```python
from build123d import *

# Parameters (mm, degrees)
CUT_EXTRUDE1_START = -3.5
CUT_EXTRUDE1_DEPTH = 3.5
SKETCH4_R          = 3.723909236
CUT_EXTRUDE2_DEPTH = 3.5
CUT_EXTRUDE2_DRAFT = -45


with BuildPart() as part:
    # Sketch2 → Revolve1 (revolve)
    with BuildSketch(Plane(origin=(0, 0, 0), x_dir=(0, 0, -1), z_dir=(1, 0, 0))):
        with BuildLine():
            Line((-11.5, 0), (-11.5, 5.604695392))
            ThreePointArc((-11.5, 5.604695392), (-11.491674324, 5.646551392), (-11.467964804, 5.682035196))
            Line((-11.467964804, 5.682035196), (-11.182035196, 5.967964804))
            ThreePointArc((-11.182035196, 5.967964804), (-11.146551392, 5.991674324), (-11.104695392, 6))
            Line((-11.104695392, 6), (-6.032804608, 6))
            ThreePointArc((-6.032804608, 6), (-5.990948608, 5.991674324), (-5.955464804, 5.967964804))
            Line((-5.955464804, 5.967964804), (-5.844535196, 5.857035196))
            ThreePointArc((-5.844535196, 5.857035196), (-5.809051392, 5.833325676), (-5.767195392, 5.825))
            Line((-5.767195392, 5.825), (-4.65, 5.825))
            ThreePointArc((-4.65, 5.825), (-4.543933983, 5.781066017), (-4.5, 5.675))
            Line((-4.5, 5.675), (-4.5, 3.85))
            ThreePointArc((-4.5, 3.85), (-4.397487373, 3.602512627), (-4.15, 3.5))
            Line((-4.15, 3.5), (10.850480947, 3.5))
            Line((10.850480947, 3.5), (11.5, 2.850480947))
            Line((11.5, 2.850480947), (11.5, 0))
            Line((11.5, 0), (-11.5, 0))
        make_face()
    revolve(axis=Axis((0, 0, -11.5), (0, 0, 1)))

    # Sketch3 → Cut-Extrude1 (cut)
    with BuildSketch(Plane.XY.offset(11.5).offset(CUT_EXTRUDE1_START)):
        Polygon((3, -1.732050808), (3, 1.732050808), (0, 3.464101615), (-3, 1.732050808), (-3, -1.732050808), (0, -3.464101615), align=None)
    extrude(amount=CUT_EXTRUDE1_DEPTH, mode=Mode.SUBTRACT)


with BuildPart() as cut_extrude2_tool:
    # Sketch4 → Cut-Extrude2 (with draft: the straight prism first)
    with BuildSketch(Plane.XY.offset(11.5)):
        Circle(SKETCH4_R)
    extrude(amount=-CUT_EXTRUDE2_DEPTH)
    # Cut-Extrude2: the draft: its side faces are tilted about the plane it starts from
    cut_extrude2_sides = [cut_extrude2_tool.faces().sort_by_distance(p)[0] for p in [
        (-3.723909236, 0, 9.75),
    ]]
    draft(cut_extrude2_sides, Plane.XY.offset(11.5), CUT_EXTRUDE2_DRAFT)


with BuildPart() as part_1:
    add(part.part)

    # Cut-Extrude2: cut by cut_extrude2_tool
    add(cut_extrude2_tool.part, mode=Mode.SUBTRACT)


solid = part_1.part
```
Read the model definition and answer for the solid it produces. Units are mm, in the model's axes. A direction names the side the tool comes from. Round coordinates to 2 decimals unless told otherwise and drop trailing zeros. Write each loop counter-clockwise with the first axis right and the second up, starting at its lowest first coordinate (ties: lowest second). Pieces come first, ordered by that corner, then holes. Notation, with made-up numbers: (-26, 6) - (-22, 6) arc R8 ccw to (-22, 20) - close; hole circle Ø1 at (81, 18.5). An arc over 180 degrees is marked (long way). Use CSV: the item, a comma, the result in double quotes.
Q1. A tool of negligible diameter and unlimited length cuts with its end or side. For faces 1 (the flat face through (1, 4, 4.5)), 2 (the flat face through (1.5, 2.6, 9.6)), 3 (the cylindrical face through (0, -6, 9)), from which of +Z, -Z, +X, -X, +Y, -Y can it reach the whole face along a straight path? Write none if from no direction.
Values:
face 1,"-Z"
face 2,"+Z"
face 3,"+Z, -Z"
Q2. Each of these flat-tipped pins is pushed along its axis until it touches: pin 1 Ø5 at (x, y) = (0, -0.5) entering from +Z; pin 2 Ø1 at (y, z) = (-1, 9) entering from +X; pin 3 Ø2 at (y, z) = (1.5, -1.5) entering from +X. Where does it stop, or does it pass through?
Values:
pin 1,"stops at z = 8"
pin 2,"stops at x = 5.98"
pin 3,"stops at x = 3.46"
Q3. Determine the mould class of faces 4 (the flat face through (1.5, -2.6, 9.6)), 5 (the flat face through (4, -1, 11.5)), 6 (the cylindrical face through (1.341, 3.233, -3.455)) for opening direction Y: +Y half, -Y half, draft (parallel to the pull), parting line (faces both ways), or undercut.
Values:
face 4,"undercut"
face 5,"draft"
face 6,"parting line"
Q4. Find section C-C, the plane z = -1. Write down the section's boundary in (x, y), then the cut area to 3 significant figures.
Values:
outline,"circle Ø7 at (0, 0)"
area,"38.5 mm²"
Q5. Find section A-A, the plane z = 9.75. Write down the section's boundary in (x, y), then the cut area to 3 significant figures.
Values:
outline,"circle Ø12 at (0, 0); hole (-3, -1.73) - (0, -3.46) - (3, -1.73) - (3, 1.73) - (0, 3.46) - (-3, 1.73) - close"
area,"81.9 mm²"
Q6. Straight lines are drawn through the part: line 1 along X through (y, z) = (0.25, 9); line 2 along Z through (x, y) = (-0.25, -5.25); line 3 along X through (y, z) = (0.5, -5.5). For each, find the intervals that lie inside material, in ascending order.
Values:
line 1,"x = -5.99 to -3, 3 to 5.99"
line 2,"z = 4.5 to 11.5"
line 3,"x = -3.46 to 3.46"
